Source: CAD feature listing. Evaluate the final solid. Frame: model axes, mm. Face numbers are marked on the shaded views. A direction names the side the tool comes from. Coordinates: 2 decimals unless noted, no trailing zeros. Write each loop counter-clockwise with the first axis right and the second up, starting at its lowest first coordinate (ties: lowest second). Pieces come first, ordered by that corner, then holes. Notation, with made-up numbers: (75, 10.5) -> (98, 10.5) arc R12 ccw to (98, 15.5) -> close; hole circle Ø8 at (49, 86.25). An arc over 180 degrees is marked (long way). Write item = value, one per line.
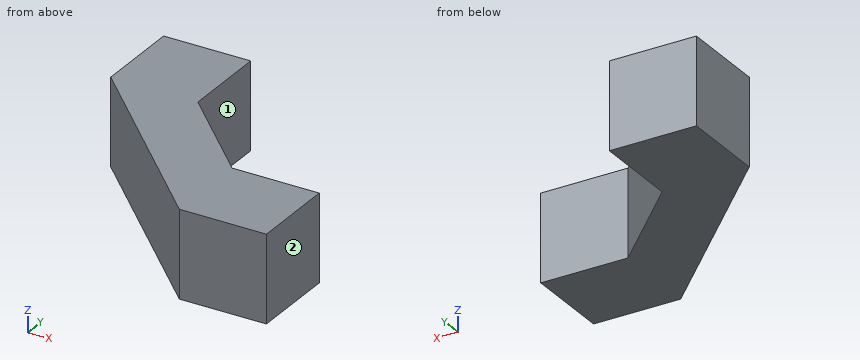
Autodesk Inventor part; units mm, degrees
ref_plane "YZ Plane" through (0, 0, 0) normal (1, 0, 0) x (0, 1, 0)
ref_plane "XZ Plane" through (0, 0, 0) normal (0, 1, 0) x (-1, 0, 0)
ref_plane "XY Plane" through (0, 0, 0) normal (0, 0, 1) x (1, 0, 0)
sketch "Sketch1" plane through (0, 0, 0) normal (0, 0, 1) x (1, 0, 0)
  line L0 (-0.0466, 4.8213) -> (-6.0466, 4.8213)
  line L1 (-6.0466, 4.8213) -> (-6.0466, 10.8213)
  line L2 (-6.0466, 10.8213) -> (-0.0466, 10.8213)
  line L3 (-0.0466, 10.8213) -> (-0.0466, 4.8213)
  line L4 (-12.0466, 16.8213) -> (-18.0466, 16.8213)
  line L5 (-18.0466, 16.8213) -> (-18.0466, 22.8213)
  line L6 (-18.0466, 22.8213) -> (-12.0466, 22.8213)
  line L7 (-12.0466, 22.8213) -> (-12.0466, 16.8213)
  line L8 (-6.0466, 10.8213) -> (-12.0466, 16.8213)
  line L9 (-6.0466, 4.8213) -> (-18.0466, 16.8213)
  point P0 (0, 0)
  dimension "d0" = 6
  dimension "d1" = 6
  dimension "d4" = 6
  dimension "d5" = 6
  dimension "d6" = 45
  dimension "d7" = 6
extrude "Extrusion1" add sketch "Sketch1" along normal blind 6
properties part number "TriangleConnector"
1) Cut plane A-A, the plane z = 5.2. Output: boundary loops of the cut face in (x, y).
Answer block:
outline = (-18.05, 16.82) -> (-6.05, 4.82) -> (-0.05, 4.82) -> (-0.05, 10.82) -> (-6.05, 10.82) -> (-12.05, 16.82) -> (-12.05, 22.82) -> (-18.05, 22.82) -> close
2) Material intervals for probe 1 along Y at (x, z) = (-3.5, 3.95); probe 2 along X at (y, z) = (18.25, 4.05); probe 3 along Y at (x, z) = (-13.75, 1.55), sorted ascending. Write a range as [from, to].
Answer block:
probe_1 = [4.82, 10.82]
probe_2 = [-18.05, -12.05]
probe_3 = [12.52, 22.82]
3) Reachability of the marked faces 1 and 2 from +Z, -Z, +X, -X, +Y, -Y: full face, straight path, thin tool, end or side. Return the list, or none.
Answer block:
face_1 = +Z, -Z, +X, +Y
face_2 = +Z, -Z, +X, +Y, -Y
4) First-contact query: pin 1 Ø3 at (y, z) = (20, 3) entering from +X; pin 2 Ø1.5 at (x, z) = (-8, 2) entering from -Y; pin 3 Ø2 at (x, z) = (-8.5, 1) entering from +Y. Flat tips, straight axial feed; report the tip coordinate or a pass-through.
Answer block:
pin_1 = -12.05
pin_2 = 6.02
pin_3 = 14.27
5) Cut plane C-C, the plane x = -15.5. Output: boundary loops of the cut face in (y, z).
Answer block:
outline = (14.27, 0) -> (22.82, 0) -> (22.82, 6) -> (14.27, 6) -> close
6) Cut plane B-B, the plane y = 20. Output: boundary loops of the cut face in (x, z).
Answer block:
outline = (-18.05, 0) -> (-12.05, 0) -> (-12.05, 6) -> (-18.05, 6) -> close
